The listing builds one solid part. Answer for the finished solid, in the listing's coordinates (mm). Face numbers are marked on the shaded views. A direction names the side the tool comes from. Coordinates: 2 decimals unless noted, no trailing zeros. Order: outer loops, then holes, each group sorted by start corner. A loop starts at its lowest first (then second) coordinate and runs counter-clockwise, first axis right, second up. Notation, with made-up numbers: (11, -7) -> (40, -7) arc R15 ccw to (40, -2) -> close; hole circle Ø9 at (-17.5, -1). An arc over 180 degrees is marked (long way). Write item = value, one per line.
Autodesk Inventor part; units mm, degrees
ref_plane "YZ Plane" through (0, 0, 0) normal (1, 0, 0) x (0, 1, 0)
ref_plane "XZ Plane" through (0, 0, 0) normal (0, 1, 0) x (-1, 0, 0)
ref_plane "XY Plane" through (0, 0, 0) normal (0, 0, 1) x (1, 0, 0)
ref_plane "Work Plane5" through (0, 3, 0) normal (0, 1, 0) x (1, 0, 0)
sketch "Sketch45" plane through (0, 3, 0) normal (0, 1, 0) x (1, 0, 0)
  line L0 (35, -20) -> (-3, -20)
  line L1 (-3, -20) -> (-3, 20)
  line L2 (-3, 20) -> (35, 20)
  line L3 (35, 20) -> (35, -20)
  point P0 (0, 0)
  dimension "d142" = 38
  dimension "d143" = 40
extrude "Extrusion34" add sketch "Sketch45" along normal blind 30
ref_plane "Work Plane2" through (0, 0, 0) normal (0, -1, 0) x (1, 0, 0)
sketch "Sketch47" plane through (0, 0, 0) normal (0, -1, 0) x (1, 0, 0)
  circle A0 centre (16, 0) radius 18
  point P0 (0, 0)
  dimension "d146" = 36
extrude "Extrusion35" cut sketch "Sketch47" against normal blind 30 draft -15
ref_plane "Work Plane1" through (0, 3, 0) normal (0, 1, 0) x (1, 0, 0)
sketch "Sketch74" plane through (0, 33, 0) normal (0, 1, 0) x (1, 0, 0)
  circle A0 centre (20, 0) radius 1.15
  point P0 (0, 0)
  dimension "d210" = 2.3
extrude "Extrusion51" cut sketch "Sketch74" against normal blind 10
sketch "Sketch77" plane through (0, 3, 0) normal (0, -1, 0) x (1, 0, 0)
  circle A0 centre (16, 0) radius 17.5
  point P0 (0, 0)
  dimension "d219" = 35
sketch "Sketch78" plane through (0, 3, 0) normal (0, -1, 0) x (1, 0, 0)
  line L0 (45, -30) -> (-13, -30)
  line L1 (-13, -30) -> (-13, 30)
  line L2 (-13, 30) -> (45, 30)
  line L3 (45, 30) -> (45, -30)
  line L4 (45, -30) -> (-13, 30) construction
  line L5 (-13, -30) -> (45, 30) construction
  point P0 (0, 0)
  point P1 (16, 0)
  dimension "d220" = 58
  dimension "d221" = 60
extrude "Extrusion53" add sketch "Sketch78" against normal blind 3
extrude "Extrusion54" cut sketch "Sketch77" against normal blind 3
sketch "Sketch81" plane through (0, 3, 0) normal (0, -1, 0) x (1, 0, 0)
  circle A0 centre (33.5, -25) radius 2.7
  line L0 (-13, -30) -> (45, -30)
  line L1 (45, -30) -> (45, 30)
  circle A1 centre (16, -25) radius 2.7
  circle A2 centre (-1.5, -25) radius 2.7
  circle A3 centre (-1.5, 25) radius 2.7
  circle A4 centre (16, 25) radius 2.7
  circle A5 centre (33.5, 25) radius 2.7
  point P0 (0, 0)
  dimension "mag_D" = 5.4
  dimension "d232" = 5
  dimension "d233" = 11.5
  dimension "d234" = 5.4
  dimension "d235" = 17.5
  dimension "d236" = 5.4
  dimension "d237" = 17.5
  dimension "d243" = 5.4
  dimension "d245" = 5.4
  dimension "d246" = 17.5
  dimension "d247" = 5.4
  dimension "d248" = 17.5
extrude "Extrusion56" cut sketch "Sketch81" against normal blind 30
sketch "Sketch83" plane through (0, 3, 0) normal (0, -1, 0) x (1, 0, 0)
  line L0 (-8.9107, -2) -> (-8.9107, 2)
  line L1 (-8.9107, 2) -> (-5.4466, 0)
  line L2 (-5.4466, 0) -> (-8.9107, -2)
  point P0 (0, 0)
  point P1 (-8.9107, -9.2159)
  point P2 (-7.756, 0)
  dimension "d253" = 4
extrude "Extrusion57" add sketch "Sketch83" along normal blind 4.5
equation "\"d234\" = mag_D"
equation "\"d236\" = mag_D"
equation "\"d237\" = d235"
equation "\"d243\" = mag_D"
equation "\"d245\" = mag_D"
equation "\"d246\" = d235"
equation "\"d247\" = mag_D"
equation "\"d248\" = d235"
properties part number "liquid_port_v05"
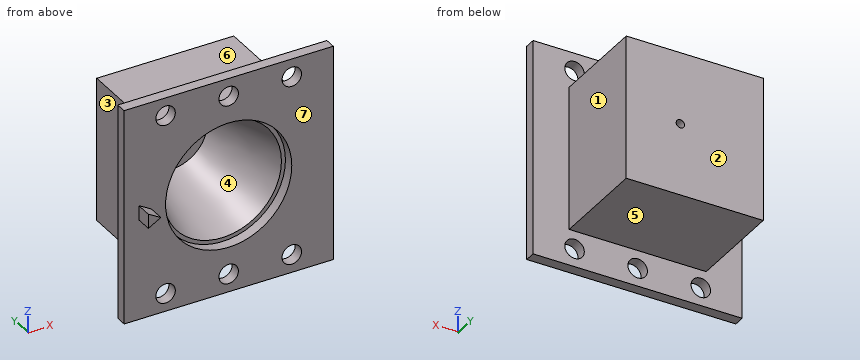
Q1. Section A-A, the plane z = -25 is taken. Give the vertices of the cut face in (x, y).
The answers:
outline = (-13, 3) -> (-4.2, 3) -> (-4.2, 6) -> (-13, 6) -> close; (1.2, 3) -> (13.3, 3) -> (13.3, 6) -> (1.2, 6) -> close; (18.7, 3) -> (30.8, 3) -> (30.8, 6) -> (18.7, 6) -> close; (36.2, 3) -> (45, 3) -> (45, 6) -> (36.2, 6) -> close
Q2. A tool of negligible diameter and unlimited length cuts with its end or side. For the marked faces 1, 2 and 3, from which of +Z, -Z, +X, -X, +Y, -Y can it reach the whole face along a straight path? Write none if from no direction.
The answers:
face_1 = +Z, -Z, +X, +Y
face_2 = +Z, -Z, +X, -X, +Y
face_3 = +Z, -Z, -X, +Y
Q3. Section B-B, the plane x = 16 is taken. Give the vertices of the cut face in (y, z), plus the area to 3 significant figures.
The answers:
outline = (3, -30) -> (6, -30) -> (6, -27.7) -> (3, -27.7) -> close; (3, -22.3) -> (6, -22.3) -> (6, -20) -> (33, -20) -> (33, 20) -> (6, 20) -> (6, 22.3) -> (3, 22.3) -> (3, 17.5) -> (6, 17.5) -> (6, 16.39) -> (30, 9.96) -> (30, -9.96) -> (6, -16.39) -> (6, -17.5) -> (3, -17.5) -> close; (3, 27.7) -> (6, 27.7) -> (6, 30) -> (3, 30) -> close
area = 490 mm2
Q4. Section C-C, the plane y = 4.5 is taken. Give the vertices of the cut face in (x, z), plus the area to 3 significant figures.
The answers:
outline = (-13, -30) -> (45, -30) -> (45, 30) -> (-13, 30) -> close; hole circle Ø5.4 at (-1.5, -25); hole circle Ø5.4 at (-1.5, 25); hole circle Ø35 at (16, 0); hole circle Ø5.4 at (16, -25); hole circle Ø5.4 at (16, 25); hole circle Ø5.4 at (33.5, -25); hole circle Ø5.4 at (33.5, 25)
area = 2,380 mm2
Q5. The mould has two halves that part along Z. Classify the marked faces 4, 5, 6 and 7: released by +Z, released by -Z, zero draft, split by the parting line, or undercut.
The answers:
face_4 = undercut
face_5 = released by -Z
face_6 = released by +Z
face_7 = zero draft
Q6. Section D-D, the plane z = 19 is taken. Give the vertices of the cut face in (x, y), plus the area to 3 significant figures.
The answers:
outline = (-13, 3) -> (45, 3) -> (45, 6) -> (35, 6) -> (35, 33) -> (-3, 33) -> (-3, 6) -> (-13, 6) -> close
area = 1,200 mm2
Q7. Each of these flat-tipped pins is pushed along its axis until it touches: pin 1 Ø6 at (x, z) = (13.5, -21) entering from +Y; pin 2 Ø3 at (x, z) = (16, 25) entering from -Y (1 decimal); pin 3 Ø6 at (x, z) = (16, -25) entering from -Y; pin 4 Ø13.5 at (x, y) = (16.5, 14) entering from +Z. Where does it stop, or does it pass through?
The answers:
pin_1 = 33
pin_2 = through
pin_3 = 3
pin_4 = 20
Q8. Find the intervals of material crossed by line 1 along Z through (x, y) = (20, 32.05); line 2 along Y through (x, z) = (40, -24); line 3 along Z through (x, y) = (32.5, 20), in increasing order.
The answers:
line_1 = -20 to -1.15, 1.15 to 20
line_2 = 3 to 6
line_3 = -20 to 20
